Work out the finished part from the listing and answer in its coordinate system (mm). Round coordinates to 2 decimals unless told otherwise and drop trailing zeros. Loops run counter-clockwise (first coordinate to the right, second up) from the corner with the lowest first, then second, coordinate; pieces in that order, holes last. Notation, with made-up numbers: (-27.75, 42.25) - (-6.75, 42.25) arc R21 ccw to (-6.75, 80.25) - close; hole circle Ø11 at (15, 4). An arc over 180 degrees is marked (long way). Return JSON: item names as keys, results as strings.
from build123d import *

# Parameters (mm, degrees)
SKETCH_1_W          = 40
SKETCH_1_H          = 20
SKETCH_1_W_2        = 38
SKETCH_1_H_2        = 18
EXTRUDE_1_DEPTH     = 910
SKETCH_2_R          = 1.6
CUT_EXTRUDE_1_DEPTH = 70
SKETCH_3_R          = 1.6
CUT_EXTRUDE_2_DEPTH = 10
CUT_EXTRUDE_4_DEPTH = 10
SKETCH_6_R          = 1.6
CUT_EXTRUDE_5_DEPTH = 912.098238391
CUT_EXTRUDE_6_REACH = 913.098


with BuildPart() as part:
    # 草图1 → 拉伸-薄壁1 (new body)
    with BuildSketch(Plane.XY):
        with Locations((-20, 10)):
            Rectangle(SKETCH_1_W, SKETCH_1_H)
        with Locations((-20, 10)):
            Rectangle(SKETCH_1_W_2, SKETCH_1_H_2, mode=Mode.SUBTRACT)
    extrude(amount=EXTRUDE_1_DEPTH)

    # 草图2 → 切除-拉伸1 (cut)
    with BuildSketch(Plane.ZY.offset(40)):
        with Locations(Location((865, 10, 0), (0, 0, 270))):
            Circle(SKETCH_2_R)
        with Locations(Location((845, 10, 0), (0, 0, 270))):
            Circle(SKETCH_2_R)
        with Locations(Location((825, 10, 0), (0, 0, 270))):
            Circle(SKETCH_2_R)
        with Locations(Location((45, 10, 0), (0, 0, 270))):
            Circle(SKETCH_2_R)
        with Locations(Location((25, 10, 0), (0, 0, 270))):
            Circle(SKETCH_2_R)
        with Locations(Location((5, 10, 0), (0, 0, 270))):
            Circle(SKETCH_2_R)
    extrude(amount=-CUT_EXTRUDE_1_DEPTH, mode=Mode.SUBTRACT)

    # 草图3 → 切除-拉伸2 (cut)
    with BuildSketch(Plane.ZY.offset(40)):
        with Locations(Location((120, 10, 0), (0, 0, 270))):
            Circle(SKETCH_3_R)
        with Locations(Location((140, 10, 0), (0, 0, 270))):
            Circle(SKETCH_3_R)
        with Locations(Location((230, 10, 0), (0, 0, 270))):
            Circle(SKETCH_3_R)
        with Locations(Location((250, 10, 0), (0, 0, 270))):
            Circle(SKETCH_3_R)
    extrude(amount=-CUT_EXTRUDE_2_DEPTH, mode=Mode.SUBTRACT)

    # 草图5 → 切除-拉伸4 (cut)
    with BuildSketch(Plane(origin=(0, 20, 0), x_dir=(1, 0, 0), z_dir=(0, 1, 0))):
        with BuildLine():
            Line((-21, -120), (-21, -140))
            ThreePointArc((-21, -140), (-28, -147), (-35, -140))
            Line((-35, -140), (-35, -120))
            ThreePointArc((-35, -120), (-28, -113), (-21, -120))
        make_face()
        with BuildLine():
            Line((-21, -230), (-21, -250))
            ThreePointArc((-21, -250), (-28, -257), (-35, -250))
            Line((-35, -250), (-35, -230))
            ThreePointArc((-35, -230), (-28, -223), (-21, -230))
        make_face()
        with BuildLine():
            Line((-21, -20), (-21, -40))
            ThreePointArc((-21, -40), (-28, -47), (-35, -40))
            Line((-35, -40), (-35, -20))
            ThreePointArc((-35, -20), (-28, -13), (-21, -20))
        make_face()
        with BuildLine():
            Line((-21, -870), (-21, -890))
            ThreePointArc((-21, -890), (-28, -897), (-35, -890))
            Line((-35, -890), (-35, -870))
            ThreePointArc((-35, -870), (-28, -863), (-21, -870))
        make_face()
    extrude(amount=-CUT_EXTRUDE_4_DEPTH, mode=Mode.SUBTRACT)

    # 草图6 → 切除-拉伸5 (cut, through all)
    with BuildSketch(Plane(origin=(0, 20, 0), x_dir=(1, 0, 0), z_dir=(0, 1, 0))):
        with Locations(Location((-30, -700, 0), (0, 0, 270))):
            Circle(SKETCH_6_R)
        with Locations(Location((-10, -700, 0), (0, 0, 270))):
            Circle(SKETCH_6_R)
        with Locations(Location((-10, -680, 0), (0, 0, 270))):
            Circle(SKETCH_6_R)
        with Locations(Location((-10, -660, 0), (0, 0, 270))):
            Circle(SKETCH_6_R)
        with Locations(Location((-10, -640, 0), (0, 0, 270))):
            Circle(SKETCH_6_R)
        with Locations(Location((-10, -620, 0), (0, 0, 270))):
            Circle(SKETCH_6_R)
        with Locations(Location((-10, -600, 0), (0, 0, 270))):
            Circle(SKETCH_6_R)
        with Locations(Location((-10, -580, 0), (0, 0, 270))):
            Circle(SKETCH_6_R)
        with Locations(Location((-10, -560, 0), (0, 0, 270))):
            Circle(SKETCH_6_R)
        with Locations(Location((-10, -540, 0), (0, 0, 270))):
            Circle(SKETCH_6_R)
        with Locations(Location((-10, -520, 0), (0, 0, 270))):
            Circle(SKETCH_6_R)
        with Locations(Location((-30, -680, 0), (0, 0, 270))):
            Circle(SKETCH_6_R)
        with Locations(Location((-30, -660, 0), (0, 0, 270))):
            Circle(SKETCH_6_R)
        with Locations(Location((-30, -640, 0), (0, 0, 270))):
            Circle(SKETCH_6_R)
        with Locations(Location((-30, -620, 0), (0, 0, 270))):
            Circle(SKETCH_6_R)
        with Locations(Location((-30, -600, 0), (0, 0, 270))):
            Circle(SKETCH_6_R)
        with Locations(Location((-30, -580, 0), (0, 0, 270))):
            Circle(SKETCH_6_R)
        with Locations(Location((-30, -560, 0), (0, 0, 270))):
            Circle(SKETCH_6_R)
        with Locations(Location((-30, -540, 0), (0, 0, 270))):
            Circle(SKETCH_6_R)
        with Locations(Location((-30, -520, 0), (0, 0, 270))):
            Circle(SKETCH_6_R)
    extrude(amount=-CUT_EXTRUDE_5_DEPTH, mode=Mode.SUBTRACT)

    # 草图7 → 切除-拉伸6 (cut, up to next)
    with BuildSketch(Plane(origin=(0, 0, 0), x_dir=(0, 0, -1), z_dir=(1, 0, 0)), mode=Mode.PRIVATE) as cut_extrude_6_sk1:
        with BuildLine():
            Line((-712, 15), (-697, 15))
            ThreePointArc((-697, 15), (-692, 10), (-697, 5))
            Line((-697, 5), (-712, 5))
            ThreePointArc((-712, 5), (-717, 10), (-712, 15))
        make_face()
    cut_extrude_6_tool1 = extrude(cut_extrude_6_sk1.sketch, amount=-CUT_EXTRUDE_6_REACH, mode=Mode.PRIVATE) & part.part
    # 草图7 → 切除-拉伸6 (cut, up to next)
    with BuildSketch(Plane(origin=(0, 0, 0), x_dir=(0, 0, -1), z_dir=(1, 0, 0)), mode=Mode.PRIVATE) as cut_extrude_6_sk2:
        with BuildLine():
            Line((-672, 15), (-657, 15))
            ThreePointArc((-657, 15), (-652, 10), (-657, 5))
            Line((-657, 5), (-672, 5))
            ThreePointArc((-672, 5), (-677, 10), (-672, 15))
        make_face()
    cut_extrude_6_tool2 = extrude(cut_extrude_6_sk2.sketch, amount=-CUT_EXTRUDE_6_REACH, mode=Mode.PRIVATE) & part.part
    # 草图7 → 切除-拉伸6 (cut, up to next)
    with BuildSketch(Plane(origin=(0, 0, 0), x_dir=(0, 0, -1), z_dir=(1, 0, 0)), mode=Mode.PRIVATE) as cut_extrude_6_sk3:
        with BuildLine():
            Line((-632, 15), (-617, 15))
            ThreePointArc((-617, 15), (-612, 10), (-617, 5))
            Line((-617, 5), (-632, 5))
            ThreePointArc((-632, 5), (-637, 10), (-632, 15))
        make_face()
    cut_extrude_6_tool3 = extrude(cut_extrude_6_sk3.sketch, amount=-CUT_EXTRUDE_6_REACH, mode=Mode.PRIVATE) & part.part
    # 草图7 → 切除-拉伸6 (cut, up to next)
    with BuildSketch(Plane(origin=(0, 0, 0), x_dir=(0, 0, -1), z_dir=(1, 0, 0)), mode=Mode.PRIVATE) as cut_extrude_6_sk4:
        with BuildLine():
            Line((-592, 15), (-577, 15))
            ThreePointArc((-577, 15), (-572, 10), (-577, 5))
            Line((-577, 5), (-592, 5))
            ThreePointArc((-592, 5), (-597, 10), (-592, 15))
        make_face()
    cut_extrude_6_tool4 = extrude(cut_extrude_6_sk4.sketch, amount=-CUT_EXTRUDE_6_REACH, mode=Mode.PRIVATE) & part.part
    # 草图7 → 切除-拉伸6 (cut, up to next)
    with BuildSketch(Plane(origin=(0, 0, 0), x_dir=(0, 0, -1), z_dir=(1, 0, 0)), mode=Mode.PRIVATE) as cut_extrude_6_sk5:
        with BuildLine():
            Line((-552, 15), (-537, 15))
            ThreePointArc((-537, 15), (-532, 10), (-537, 5))
            Line((-537, 5), (-552, 5))
            ThreePointArc((-552, 5), (-557, 10), (-552, 15))
        make_face()
    cut_extrude_6_tool5 = extrude(cut_extrude_6_sk5.sketch, amount=-CUT_EXTRUDE_6_REACH, mode=Mode.PRIVATE) & part.part
    add(cut_extrude_6_tool1.solids().sort_by_distance((0, 10, 704.5))[0], mode=Mode.SUBTRACT)
    add(cut_extrude_6_tool2.solids().sort_by_distance((0, 10, 664.5))[0], mode=Mode.SUBTRACT)
    add(cut_extrude_6_tool3.solids().sort_by_distance((0, 10, 624.5))[0], mode=Mode.SUBTRACT)
    add(cut_extrude_6_tool4.solids().sort_by_distance((0, 10, 584.5))[0], mode=Mode.SUBTRACT)
    add(cut_extrude_6_tool5.solids().sort_by_distance((0, 10, 544.5))[0], mode=Mode.SUBTRACT)


solid = part.part
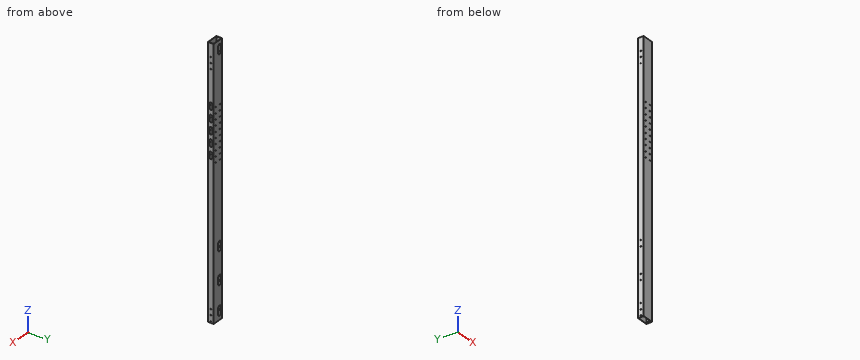
1) A flat-ended cylindrical pin translates along its axis: pin 1 (3 mm diameter, centred on x = -30, z = 660, fed in from +Y). Find the tip coordinate at first contact, or state that the pin passes through.
Verdict:
{"pin 1": "passes through"}
2) Find the intervals of material crossed by L1, parallel to X at y = 0.4, z = 540; L2, parallel to Y at x = -10, z = 254; L3, parallel to X at y = 1.5, z = 558.5, in increasing order.
Verdict:
{"L1": "x = -40 to -31.6, -28.4 to -11.6, -8.4 to 0", "L2": "y = 0 to 1, 19 to 20", "L3": "x = -40 to -39, -1 to 0"}
3) Section A-A (z = 480.5) is taken. Give the vertices of the cut face in (x, y), and give its area (3 significant figures).
Verdict:
{"outline": "(-40, 0) - (0, 0) - (0, 20) - (-40, 20) - close; hole (-39, 1) - (-1, 1) - (-1, 19) - (-39, 19) - close", "area": "116 mm2"}
